Design review of the part built by this model. Coordinates are the model's own, in mm. A direction names the side the tool comes from. Coordinates: 2 decimals unless noted, no trailing zeros. Loops run counter-clockwise (first coordinate to the right, second up) from the corner with the lowest first, then second, coordinate; pieces in that order, holes last. Notation, with made-up numbers: M -0.5,57 L 50.5,57 A18 cw 50.5,67 Z; hole C -29,-3 d8. An arc over 180 degrees is marked long. Write item = value, one per line. Start each with the question number.
```python
from build123d import *

# Parameters (mm, degrees)
F5_DEPTH      = 150
F5_DEPTH_BACK = 150
F6_W          = 12.5
F6_H          = 300
F7_DEPTH      = 15
F9_W          = 30
F9_H          = 30
F10_DEPTH     = 15


with BuildPart() as f5:
    # F2 (on Front) → F5 (new body, two sides)
    with BuildSketch(Plane.XZ) as f5_sk:
        Polygon((-100, 300), (-100, 0), (-85, 15), (-85, 285), align=None)
    extrude(amount=-F5_DEPTH)
    extrude(f5_sk.sketch, amount=F5_DEPTH_BACK)

    # F6 (on offset) → F7 (cut)
    with BuildSketch(Plane.XZ.offset(-150)):
        with Locations((-86.25, 150)):
            Rectangle(F6_W, F6_H)
    extrude(amount=F7_DEPTH, mode=Mode.SUBTRACT)

    # F9 (on offset) → F10 (join)
    with BuildSketch(Plane.XZ.offset(-135)):
        with Locations((-70, 270)):
            Rectangle(F9_W, F9_H)
        with Locations((-70, 30)):
            Rectangle(F9_W, F9_H)
    extrude(amount=F10_DEPTH)


solid = f5.part
```
(1) Insertion check: pin 1 (6 mm diameter, centred on x = -90.5, y = -61.5, fed in from -Z); pin 2 (12 mm diameter, centred on y = 140.5, z = 153.5, fed in from +X); pin 3 (12 mm diameter, centred on x = -76, y = -72.5, fed in from +Z); pin 4 (9 mm diameter, centred on x = -65.5, z = 268.5, fed in from -Y). Each pin has a flat end and moves straight along its axis. Give the tip position at first contact, or say it passes through.
(2) Take a section at B-B (y = 126). State the section outline as (x, z) points, plus the area to 4 significant figures.
(3) Take a section at A-A (x = -75). State the section outline as (y, z) points.
(4) Take a section at D-D (y = -106). State the section outline as (x, z) points.
(5) Take a section at C-C (z = 120.5). State the section outline as (x, y) points.
(6) To check wall thickness, follow L1, parallel to Y at x = -85.5, z = 183.5; L2, parallel to X at y = -57.5, z = 206.5; L3, parallel to Z at x = -94, y = -22. State the ranges of each line that lie inside material, in increasing order.
(7) Tool access review of faces 1 (the flat face through (-70, 128, 285)), 2 (the flat face through (-70, 120, 30)), 3 (the flat face through (-70, 128, 255)), 4 (the flat face through (-87, 135, 152)): name each direction out of +Z, -Z, +X, -X, +Y, -Y from which nothing blocks a thin tool from reaching the whole face with its end or side.
Results list:
q1.pin_1 = 6.5
q1.pin_2 = -85
q1.pin_3 = through
q1.pin_4 = 120
q2.outline = M -100,0 L -85,15 L -55,15 L -55,45 L -85,45 L -85,255 L -55,255 L -55,285 L -85,285 L -100,300 Z
q2.area = 6,075 mm^2
q3.outline = M 120,15 L 135,15 L 135,45 L 120,45 Z; M 120,255 L 135,255 L 135,285 L 120,285 Z
q4.outline = M -100,0 L -85,15 L -85,285 L -100,300 Z
q5.outline = M -100,-150 L -85,-150 L -85,135 L -92.5,135 L -92.5,150 L -100,150 Z
q6.L1 = -150 to 135
q6.L2 = -100 to -85
q6.L3 = 6 to 294
q7.face_1 = +Z, +X, +Y, -Y
q7.face_2 = +Z, -Z, +X, -Y
q7.face_3 = +X, +Y, -Y
q7.face_4 = +Z, -Z, +X, +Y
